Verification items for the finished model (mm, model axes). Round coordinates to 2 decimals unless told otherwise and drop trailing zeros. Write each loop counter-clockwise with the first axis right and the second up, starting at its lowest first coordinate (ties: lowest second). Pieces come first, ordered by that corner, then holes.
from build123d import *

# Parameters (mm, degrees)
MODEL_R                 = 1.5
SALIENTE_EXTRUIR1_DEPTH = 3


with BuildPart() as part:
    # Model → Saliente-Extruir1 (new body)
    with BuildSketch(Plane.XY):
        with BuildLine():
            Line((145.837507261, 264.056255289), (162.519487777, 247.374274774))
            ThreePointArc((162.519487777, 247.374274774), (168.883448807, 247.374274774), (168.883448807, 253.738235805))
            Line((168.883448807, 253.738235805), (150.883448807, 271.738235805))
            ThreePointArc((150.883448807, 271.738235805), (149.423543738, 272.713713186), (147.701468292, 273.056255289))
            Line((147.701468292, 273.056255289), (120.601468292, 273.056255289))
            ThreePointArc((120.601468292, 273.056255289), (117.490198455, 271.767525127), (116.201468292, 268.656255289))
            Line((116.201468292, 268.656255289), (116.201468292, 268.456255289))
            ThreePointArc((116.201468292, 268.456255289), (117.490198455, 265.344985452), (120.601468292, 264.056255289))
            Line((120.601468292, 264.056255289), (145.837507261, 264.056255289))
        make_face()
        with Locations((129.701468292, 268.556255289)):
            Circle(MODEL_R, mode=Mode.SUBTRACT)
        with Locations((138.701468292, 268.556255289)):
            Circle(MODEL_R, mode=Mode.SUBTRACT)
        with Locations((120.701468292, 268.556255289)):
            Circle(MODEL_R, mode=Mode.SUBTRACT)
        with Locations((147.701468292, 268.556255289)):
            Circle(MODEL_R, mode=Mode.SUBTRACT)
        with Locations((165.701468292, 250.556255289)):
            Circle(MODEL_R, mode=Mode.SUBTRACT)
        with Locations((156.701468292, 259.556255289)):
            Circle(MODEL_R, mode=Mode.SUBTRACT)
    extrude(amount=SALIENTE_EXTRUIR1_DEPTH)


solid = part.part
Q1. Sectioned sample at B-B (x = 165). Enter the section's corners in (y, z), plus the area to 3 significant figures.
Recorded:
outline: (246.11, 0) - (249.23, 0) - (249.23, 3) - (246.11, 3) - close; (251.88, 0) - (257.62, 0) - (257.62, 3) - (251.88, 3) - close
area: 26.6 mm2
Q2. Sectioned sample at D-D (x = 127). Enter the section's corners in (y, z).
Recorded:
outline: (264.06, 0) - (273.06, 0) - (273.06, 3) - (264.06, 3) - close
Q3. Depth check by flat-ended pin: P1, Ø1.5, axis at x = 134, z = 1.5, coming from the -Y side; P2, Ø1, axis at x = 147.5, z = 2.5, coming from the -Y side. Enter the tip coordinate at first touch or a pass-through.
Recorded:
P1: stops at y = 264.06
P2: stops at y = 261.89
Q4. Release check for a two-part mould opening along X. For faces 1 (the flat face through (133, 264.056, 1)), 2 (the cylindrical face through (119.596, 269.57, 1.479)), 3 (the cylindrical face through (117.456, 265.379, 1.479)) record: released by +X, released by -X, zero draft, split by the parting line, or undercut.
Recorded:
face 1: zero draft
face 2: undercut
face 3: released by -X
Q5. Sectioned sample at C-C (z = 2.35). Enter the section's corners in (x, y), plus the area to 3 significant figures.
Recorded:
outline: (116.2, 268.46) arc R4.4 ccw to (120.6, 264.06) - (145.84, 264.06) - (162.52, 247.37) arc R4.5 ccw to (168.88, 253.74) - (150.88, 271.74) arc R4.5 ccw to (147.7, 273.06) - (120.6, 273.06) arc R4.4 ccw to (116.2, 268.66) - close; hole circle Ø3 at (120.7, 268.56); hole circle Ø3 at (129.7, 268.56); hole circle Ø3 at (138.7, 268.56); hole circle Ø3 at (147.7, 268.56); hole circle Ø3 at (156.7, 259.56); hole circle Ø3 at (165.7, 250.56)
area: 493 mm2
Q6. Material ranges on line 1 along X through (y, z) = (267.25, 0.7); line 2 along Y through (x, z) = (140.5, 0.7); line 3 along X through (y, z) = (250.5, 2.15), recorded low to high.
Recorded:
line 1: x = 116.37 to 119.96, 121.44 to 128.96, 130.44 to 137.96, 139.44 to 146.96, 148.44 to 155.37
line 2: y = 264.06 to 273.06
line 3: x = 159.39 to 164.2, 167.2 to 170.2
Q7. Sectioned sample at A-A (y = 267.75). Enter the section's corners in (x, z).
Recorded:
outline: (116.26, 0) - (119.44, 0) - (119.44, 3) - (116.26, 3) - close; (121.97, 0) - (128.44, 0) - (128.44, 3) - (121.97, 3) - close; (130.97, 0) - (137.44, 0) - (137.44, 3) - (130.97, 3) - close; (139.97, 0) - (146.44, 0) - (146.44, 3) - (139.97, 3) - close; (148.97, 0) - (154.87, 0) - (154.87, 3) - (148.97, 3) - close
